Source: three-view drawing plus pictorial views. Frame: mm from the lowest corner of the part. A direction names the side the tool comes from. Coordinates: 2 decimals unless noted, no trailing zeros. Order: outer loops, then holes, each group sorted by start corner. A loop starts at its lowest first (then second) coordinate and runs counter-clockwise, first axis right, second up. Notation, with made-up numbers: M -40,-31.75 L 11,-31.75 A10 ccw 11,-23.75 Z; hole C 72,1.5 d9. An arc over 180 degrees is marked long. Use CSV: the item, a comma, the result in double quotes. Start each with the question number.
Q1. Access query for the marked faces 1, 2 and 3. Directions: +Z, -Z, +X, -X, +Y, -Y. A direction counts if a zero-diameter tool reaches every point of the face in a straight line with its end or side. Return the directions, or none.
Q2. Section query D-D, the plane y = 11. Output: boundary loops of the cut face in (x, z), and give its area (4 significant figures).
Q3. Section query B-B, the plane x = 109.5. Output: boundary loops of the cut face in (y, z).
Q4. Section query C-C, the plane x = 43. Output: boundary loops of the cut face in (y, z) (1 decimal), and give its area (3 significant figures).
Q5. First-contact query: P1, Ø6, axis at y = 43.5, z = 34.5, coming from the +X side; P2, Ø6, axis at x = 184, y = 92, coming from the -Z side; P3, Ø10, axis at x = 29, z = 61, coming from the +Y side; P4, Ø6, axis at y = 87, z = 32, coming from the +X side (1 decimal). Flat tips, straight axial feed; report the tip coordinate or a pass-through.
Q6. Ray query, probe 1 along Z at (x, y) = (163.5, 84.5); probe 2 along Y at (x, z) = (44, 65.5) (1 decimal); probe 3 along X at (y, z) = (16, 42.5) (1 decimal). Return the intervals inside material, ascending.
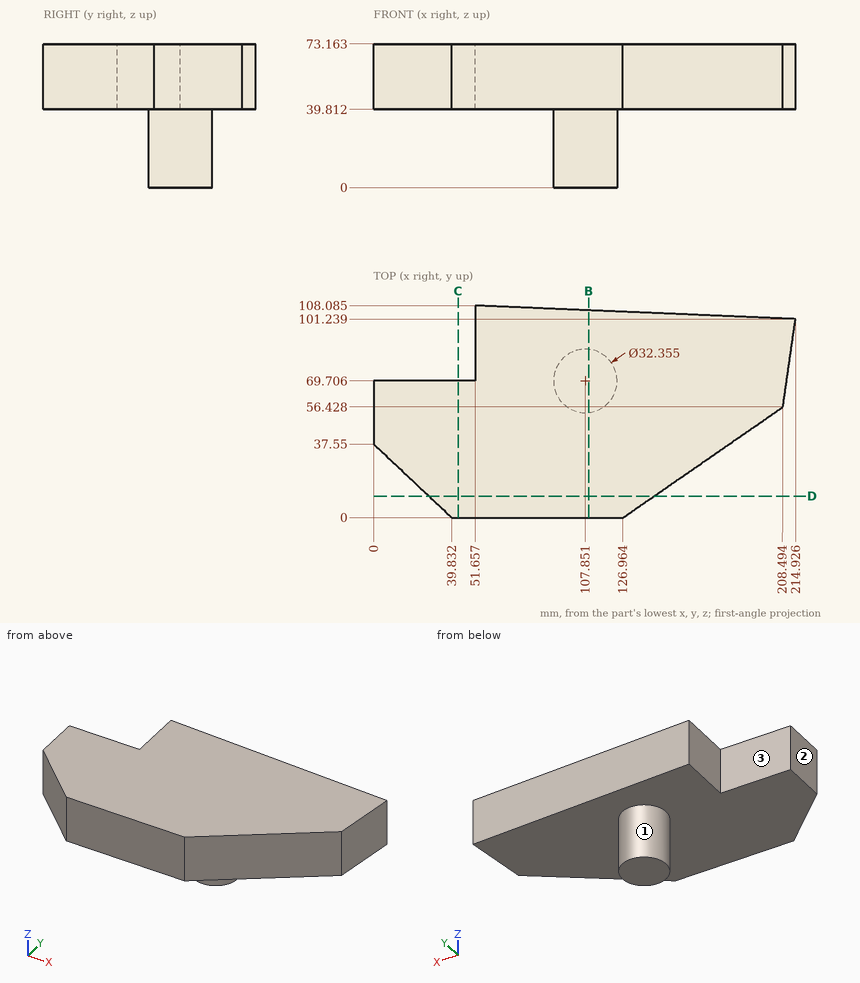
Responses:
1,face 1,"-Z"
1,face 2,"+Z, -Z, -X, +Y, -Y"
1,face 3,"+Z, -Z, -X, +Y"
2,outline,"M 28.16,39.81 L 142.86,39.81 L 142.86,73.16 L 28.16,73.16 Z"
2,area,"3,825 mm²"
3,outline,"M 0,39.81 L 53.61,39.81 L 53.61,0 L 85.8,0 L 85.8,39.81 L 105.66,39.81 L 105.66,73.16 L 0,73.16 Z"
4,outline,"M 0,39.8 L 69.7,39.8 L 69.7,73.2 L 0,73.2 Z"
4,area,"2,320 mm²"
5,P1,"passes through"
5,P2,"stops at z = 39.81"
5,P3,"stops at y = 69.71"
5,P4,"stops at x = 115.4"
6,probe 1,"z = 39.81 to 73.16"
6,probe 2,"y = 0 to 69.7"
6,probe 3,"x = 22.9 to 150.1"
